The model under review builds one solid part; all positions refer to its coordinate system, in mm. A direction names the side the tool comes from. Round coordinates to 2 decimals unless told otherwise and drop trailing zeros. Order: outer loops, then holes, each group sorted by start corner. A loop starts at its lowest first (then second) coordinate and runs counter-clockwise, first axis right, second up. Notation, with made-up numbers: M -29,-0.5 L 12,-0.5 A31 ccw 12,28.5 Z; hole C -20,67 d11. An arc over 180 degrees is marked long. Answer as a JSON object with one key per item and string values. Group by question number.
1) The part is to be moulded in two halves that separate along Z. For faces 3 (the cylindrical face through (25, 0, 44)), 4 (the flat face through (-6.4, 0.2, 10)), 5 (the flat face through (-30, 0, 25)), say which applies: +Z half, -Z half, draft (parallel to the pull), parting line (faces both ways), or undercut.
2) Consider section D-D, the plane y = -2. Write out the cut boundary in (x, z), then the cut area to 3 significant figures.
3) For faces 1 (the flat face through (25, 0, 50)), 2 (the cylindrical face through (18.289, 0.175, 11.804)), list the 3-axis set-ups (+Z, -Z, +X, -X, +Y, -Y) from which the entire face can be reached by the end or side of a thin tool; tool diameter is ignored.
4) To check wall thickness, follow line 1 (X direction, y = -9, z = 24); line 2 (Y direction, x = 0, z = 2.5); line 3 (X direction, y = 0.5, z = 12.5). State the ranges of each line that lie inside material, in increasing order.
5) Insertion check: pin 1 Ø14 at (x, y) = (0, 0) entering from +Z. The pin has a flat end and moves straight along its axis. Give the tip position at first contact, or say it passes through.
6) Consider section A-A, the plane z = 38. Write out the cut boundary in (x, y), then the cut area to 3 significant figures.
7) Consider section C-C, the plane x = 0. Write out the cut boundary in (y, z), then the cut area to 3 significant figures.
8) Consider section B-B, the plane z = 28.5. Write out the cut boundary in (x, y).
```python
from build123d import *

# Parameters (mm, degrees)
SZKIC1_W                    = 60
SZKIC1_H                    = 25
SZKIC1_R                    = 6
DODANIE_WYCI_GNI_CIE1_DEPTH = 10
SZKIC2_W                    = 10
SZKIC2_H                    = 25
DODANIE_WYCI_GNI_CIE2_DEPTH = 40
ZAOKR_GLENIE1_R             = 6
SZKIC3_R                    = 6
WYTNIJ_WYCI_GNI_CIE1_DEPTH  = 70


with BuildPart() as part:
    # Szkic1 → Dodanie-wyciągnięcie1 (new body)
    with BuildSketch(Plane.XY):
        Rectangle(SZKIC1_W, SZKIC1_H)
        Circle(SZKIC1_R, mode=Mode.SUBTRACT)
    extrude(amount=DODANIE_WYCI_GNI_CIE1_DEPTH)

    # Szkic2 → Dodanie-wyciągnięcie2 (add)
    with BuildSketch(Plane.XY.offset(10)):
        with Locations((-25, 0)):
            Rectangle(SZKIC2_W, SZKIC2_H)
        with Locations((25, 0)):
            Rectangle(SZKIC2_W, SZKIC2_H)
    extrude(amount=DODANIE_WYCI_GNI_CIE2_DEPTH)

    # Zaokrąglenie1
    zaokr_glenie1_edges = [part.edges().sort_by_distance(p)[0] for p in [
        (-20, 0, 10),
        (20, 0, 10),
    ]]
    fillet(zaokr_glenie1_edges, radius=ZAOKR_GLENIE1_R)

    # Szkic3 → Wytnij-wyciągnięcie1 (cut)
    with BuildSketch(Plane.ZY.offset(30)):
        with Locations(Location((38, 0, 0), (0, 0, 180))):
            Circle(SZKIC3_R)
    extrude(amount=-WYTNIJ_WYCI_GNI_CIE1_DEPTH, mode=Mode.SUBTRACT)


solid = part.part
```
Results list:
{
 "1": {"face 3": "undercut", "face 4": "+Z half", "face 5": "draft"},
 "2": {"outline": "M -30,0 L -5.66,0 L -5.66,10 L -14,10 A6 cw -20,16 L -20,32.34 L -30,32.34 Z; M -30,43.66 L -20,43.66 L -20,50 L -30,50 Z; M 5.66,0 L 30,0 L 30,32.34 L 20,32.34 L 20,16 A6 cw 14,10 L 5.66,10 Z; M 20,43.66 L 30,43.66 L 30,50 L 20,50 Z", "area": "1,080 mm^2"},
 "3": {"face 1": "+Z, +X, -X, +Y, -Y", "face 2": "+Z, +Y, -Y"},
 "4": {"line 1": "-30 to -20, 20 to 30", "line 2": "-12.5 to -6, 6 to 12.5", "line 3": "-30 to -18.87, 18.87 to 30"},
 "5": {"pin 1": "z = 10"},
 "6": {"outline": "M -30,-12.5 L -20,-12.5 L -20,-6 L -30,-6 Z; M -30,6 L -20,6 L -20,12.5 L -30,12.5 Z; M 20,-12.5 L 30,-12.5 L 30,-6 L 20,-6 Z; M 20,6 L 30,6 L 30,12.5 L 20,12.5 Z", "area": "260 mm^2"},
 "7": {"outline": "M -12.5,0 L -6,0 L -6,10 L -12.5,10 Z; M 6,0 L 12.5,0 L 12.5,10 L 6,10 Z", "area": "130 mm^2"},
 "8": {"outline": "M -30,-12.5 L -20,-12.5 L -20,12.5 L -30,12.5 Z; M 20,-12.5 L 30,-12.5 L 30,12.5 L 20,12.5 Z"}
}
